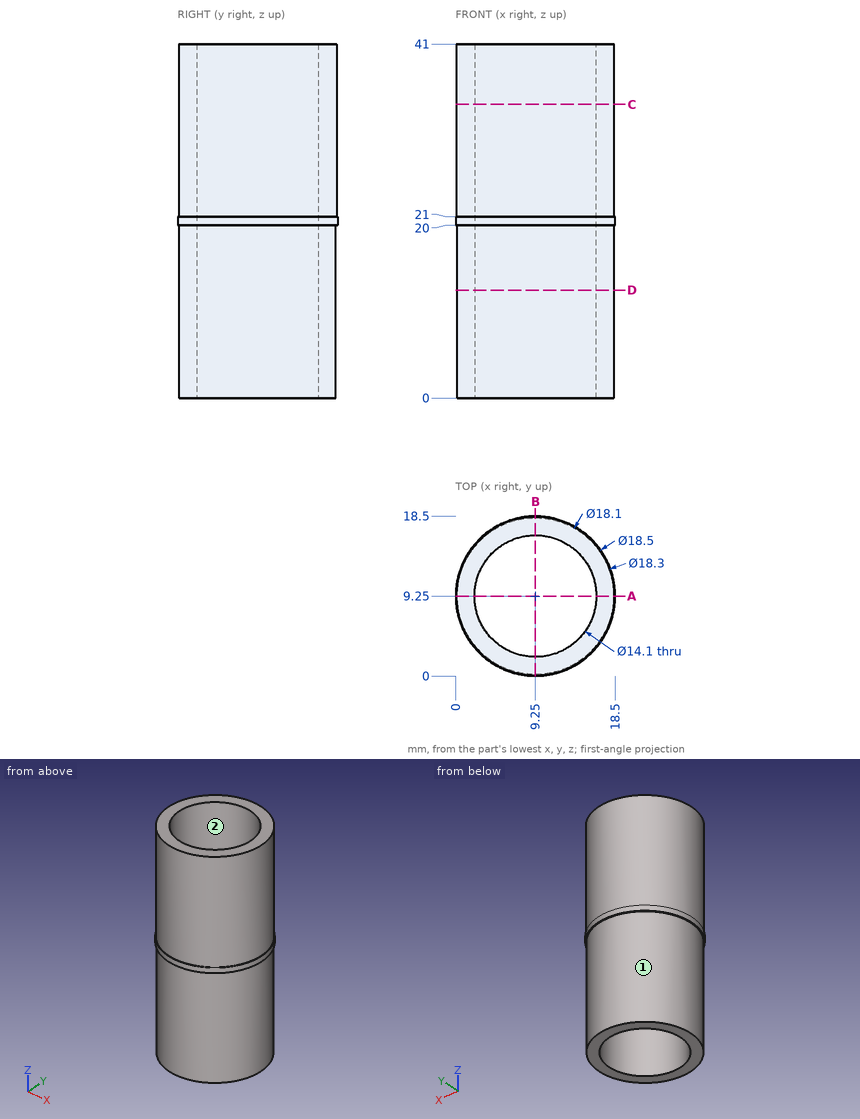
Study the drawing (mm; zero at the part's minimum x, y, z) and answer. Give positions to 0.01 mm unless a question says otherwise; leave off trailing zeros. Write each loop counter-clockwise with the first axis right and the second up, starting at its lowest first coordinate (ties: lowest second). Pieces come first, ordered by that corner, then holes.
Item 1: Find the intervals of material crossed by line 1 along Y through (x, z) = (9.25, 14); line 2 along Y through (x, z) = (9.25, 24), in increasing order.
Item 2: Section C-C, the plane z = 34 is taken. Write down the section's boundary in (x, y), plus the area to 3 significant figures.
Item 3: Section A-A, the plane y = 9.25 is taken. Write down the section's boundary in (x, z), plus the area to 3 significant figures.
Item 4: Flat-ended cylindrical pins translate along their axes: P1, Ø2, axis at x = 3.5, z = 20, coming from the +Y side; P2, Ø6, axis at y = 8.5, z = 8.5, coming from the -X side; P3, Ø2, axis at y = 9.5, z = 11, coming from the +X side. Find the tip coordinate at first contact, or state that the pin passes through.
Item 5: Determine the mould class of the marked faces 1 and 2 for opening direction X: released by +X, released by -X, zero draft, split by the parting line, or undercut.
Item 6: Section D-D, the plane z = 12.5 is taken. Write down the section's boundary in (x, y).
Completed:
1. line 1: y = 0.2 to 2.2, 16.3 to 18.3
1. line 2: y = 0.1 to 2.2, 16.3 to 18.4
2. outline: circle Ø18.3 at (9.25, 9.25); hole circle Ø14.1 at (9.25, 9.25)
2. area: 107 mm2
3. outline: (0, 20) - (0.2, 20) - (0.2, 0) - (2.2, 0) - (2.2, 41) - (0.1, 41) - (0.1, 21) - (0, 21) - close; (16.3, 0) - (18.3, 0) - (18.3, 20) - (18.5, 20) - (18.5, 21) - (18.4, 21) - (18.4, 41) - (16.3, 41) - close
3. area: 168 mm2
4. P1: stops at y = 17.19
4. P2: stops at x = 0.2
4. P3: stops at x = 18.3
5. face 1: split by the parting line
5. face 2: undercut
6. outline: circle Ø18.1 at (9.25, 9.25); hole circle Ø14.1 at (9.25, 9.25)
